Design review of the part shown in the three views and the two pictorial views. Dimensions are in mm from the part's minimum x, y and z. A direction names the side the tool comes from. Give positions to 0.01 mm unless a question says otherwise; leave off trailing zeros. Loops run counter-clockwise (first coordinate to the right, second up) from the corner with the lowest first, then second, coordinate; pieces in that order, holes last. Notation, with made-up numbers: (33, 1) -> (73, 1) arc R10 cw to (73, 8) -> close; hole circle Ø8 at (21, 79.25). An arc over 180 degrees is marked (long way). Answer as CSV lines item,"result".
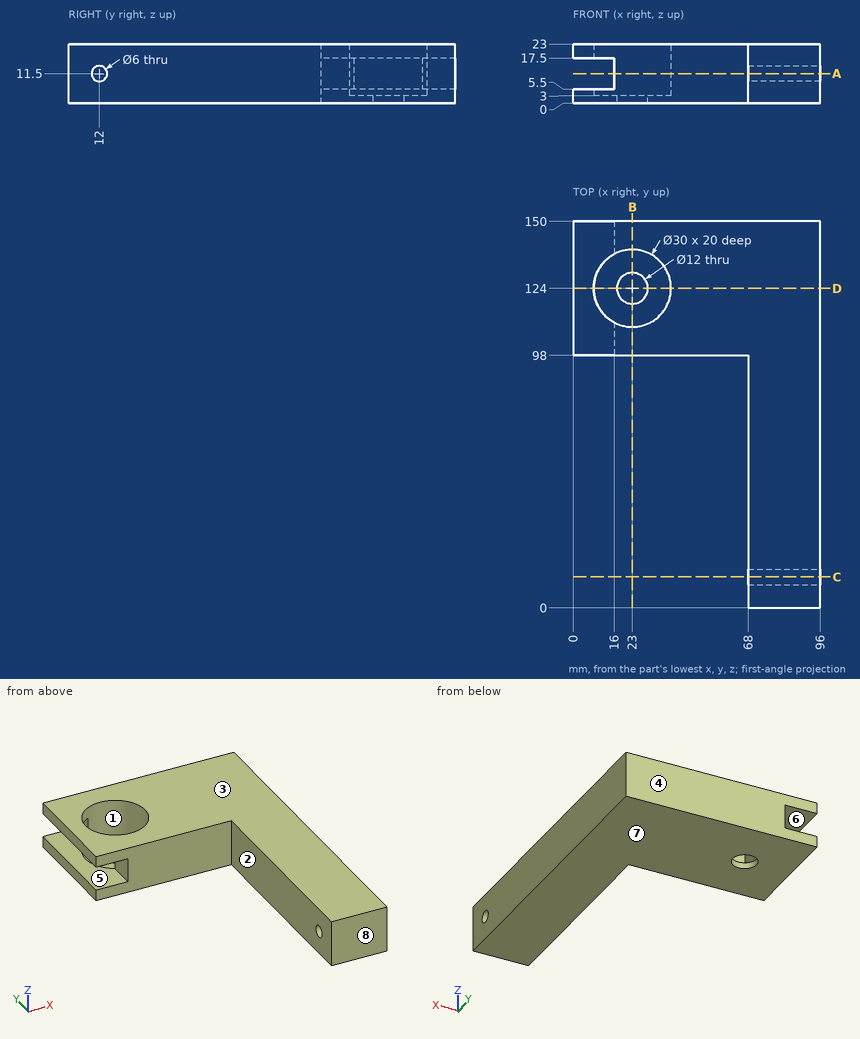
Q1. Clearance check with flat-ended pins moving along their axes: pin 1 Ø5 at (y, z) = (28.5, 20) entering from -X; pin 2 Ø3.5 at (y, z) = (143, 9.5) entering from -X; pin 3 Ø12 at (x, z) = (55.5, 18.5) entering from -Y; pin 4 Ø5.5 at (y, z) = (12, 11.5) entering from +X. State where each tip first meets the part, or that it passes through.
Filled sheet:
pin 1,"stops at x = 68"
pin 2,"stops at x = 16"
pin 3,"stops at y = 98"
pin 4,"passes through"
Q2. To check wall thickness, follow probe 1 along Y at (x, z) = (85.75, 11.5); probe 2 along Y at (x, z) = (30, 5.5); probe 3 along Y at (x, z) = (66, 18). State the ranges of each line that lie inside material, in increasing order. Write a range as from..to.
Filled sheet:
probe 1,"y = 0..9, 15..150"
probe 2,"y = 98..110.73, 137.27..150"
probe 3,"y = 98..150"
Q3. We need section B-B, the plane x = 23. State the section outline as (y, z) points, and give its area (3 significant figures).
Filled sheet:
outline,"(98, 0) -> (118, 0) -> (118, 3) -> (109, 3) -> (109, 23) -> (98, 23) -> close; (130, 0) -> (150, 0) -> (150, 23) -> (139, 23) -> (139, 3) -> (130, 3) -> close"
area,"560 mm^2"
Q4. We need section A-A, the plane z = 11.5. State the section outline as (x, y) points, and give its area (3 significant figures).
Filled sheet:
outline,"(16, 98) -> (68, 98) -> (68, 15) -> (96, 15) -> (96, 150) -> (16, 150) -> (16, 137.27) arc R15 cw (long way) to (16, 110.73) -> close; (68, 0) -> (96, 0) -> (96, 9) -> (68, 9) -> close"
area,"6,180 mm^2"
Q5. We need section D-D, the plane y = 124. State the section outline as (x, z) points.
Filled sheet:
outline,"(0, 0) -> (17, 0) -> (17, 3) -> (8, 3) -> (8, 5.5) -> (0, 5.5) -> close; (0, 17.5) -> (8, 17.5) -> (8, 23) -> (0, 23) -> close; (29, 0) -> (96, 0) -> (96, 23) -> (38, 23) -> (38, 3) -> (29, 3) -> close"
Q6. The part is to be moulded in two halves that separate along Z. For the marked faces 6, 7 and 8, say which applies: pulls with the +Z half, pulls with the -Z half, needs draft (parallel to the pull), parting line crosses it, or undercut.
Filled sheet:
face 6,"undercut"
face 7,"pulls with the -Z half"
face 8,"needs draft"
Q7. We need section C-C, the plane y = 12. State the section outline as (x, z) points, and give its area (3 significant figures).
Filled sheet:
outline,"(68, 0) -> (96, 0) -> (96, 8.5) -> (68, 8.5) -> close; (68, 14.5) -> (96, 14.5) -> (96, 23) -> (68, 23) -> close"
area,"476 mm^2"
Q8. For the marked faces 1, 2, 3, 4 and 5, list the 3-axis set-ups (+Z, -Z, +X, -X, +Y, -Y) from which the entire face can be reached by the end or side of a thin tool; tool diameter is ignored.
Filled sheet:
face 1,"+Z"
face 2,"+Z, -Z, -X, -Y"
face 3,"+Z, +X, -X, +Y, -Y"
face 4,"+Z, -Z, +X, -X, +Y"
face 5,"-X, +Y, -Y"
